Solid Edge part; units mm, degrees
sketch "Sketch1" plane through (0, 0, 0) normal (0, 0, 1) x (1, 0, 0)
  circle A0 centre (0, 0) radius 7.239
extrude "Protrusion1" add sketch "Sketch1" along normal blind 2.794
sketch "Sketch2" plane through (0, 0, 0) normal (0, 0, -1) x (1, 0, 0)
  line L0 (4.4626, 4.4626) -> (1.6334, 6.096)
  line L1 (1.6334, 6.096) -> (-1.6334, 6.096)
  line L2 (-1.6334, 6.096) -> (-4.4626, 4.4626)
  line L3 (-4.4626, 4.4626) -> (-6.096, 1.6334)
  line L4 (-6.096, 1.6334) -> (-6.096, -1.6334)
  line L5 (-6.096, -1.6334) -> (-4.4626, -4.4626)
  line L6 (-4.4626, -4.4626) -> (-1.6334, -6.096)
  line L7 (-1.6334, -6.096) -> (1.6334, -6.096)
  line L8 (1.6334, -6.096) -> (4.4626, -4.4626)
  line L9 (4.4626, -4.4626) -> (6.096, -1.6334)
  line L10 (6.096, -1.6334) -> (6.096, 1.6334)
  line L11 (6.096, 1.6334) -> (4.4626, 4.4626)
extrude "ExtrudedProtrusion_2" add sketch "Sketch2" along normal blind 10.922
sketch "Sketch3" plane through (0, 0, -10.922) normal (0, 0, -1) x (0.5, 0.866, 0)
  circle A0 centre (0, 0) radius 5.461
extrude "ExtrudedProtrusion_3" add sketch "Sketch3" along normal blind 10.16
sketch "Sketch4" plane through (0, 0, -21.082) normal (0, 0, -1) x (0, 1, 0)
  circle A0 centre (0, 0) radius 1.4
extrude "ExtrudedCutout_1" cut sketch "Sketch4" against normal blind 1.7575
Part model, mm, in its own coordinate system. A direction names the side the tool comes from. Coordinates: 2 decimals unless noted, no trailing zeros. Loops run counter-clockwise (first coordinate to the right, second up) from the corner with the lowest first, then second, coordinate; pieces in that order, holes last. Notation, with made-up numbers: (45, 87) -> (101, 87) arc R22 cw to (101, 110) -> close; hole circle Ø7 at (11.5, 57). An arc over 180 degrees is marked (long way). Use a Markdown table: item, result. Add a question column.
Item 1: Band-saw the part on C-C on z = 1. Write the cut outline in (x, y).
Item 2: Band-saw the part on D-D on y = -2.25. Write the cut outline in (x, z).
Item 3: Which spindle directions (+Z, -Z, +X, -X, +Y, -Y) get a long thin tool onto all of the face, cutting with end or side? Do faces 5 (the flat face through (-5.268, -3.068, -5.385)), 6 (the flat face through (-3.068, 5.268, -5.385)), 7 (the flat face through (0, 0, -19.324)). Say none if no direction does.
Item 4: Probe probe 1 along Z at (x, y) = (3.25, 4.75); probe 2 along Y at (x, z) = (1.5, -1.75). List the from-to ranges inside material, lowest first.
Item 5: Band-saw the part on A-A on x = 0. Write the cut outline in (y, z).
Item 6: Flat gauge pins, fed straight in: P1, Ø3.5, axis at x = -0.5, z = -7.5, coming from the +Y side; P2, Ø2.5, axis at y = -0.5, z = -5, coming from the -X side; P3, Ø3.5, axis at x = 0.5, z = -3, coming from the -Y side. Where does each tip first touch, or does it go through?
Item 7: Pull direction X, two halves, no side cores. Call faces 1 (the flat face through (-6.096, 0, -5)), 2 (the cylindrical face through (0.06, -1.4, -20.22)), 3 (the flat face through (3.03, 5.29, -5.38)), 4 (the flat face through (-1.1, -1.1, -21.082)): +X half, -X half, draft (parallel to the pull), parting line (faces both ways), or undercut.
Geometry says:
| question | item | result |
|---|---|---|
| 1 | outline | circle Ø14.48 at (0, 0) |
| 2 | outline | (-6.88, 0) -> (-5.74, 0) -> (-5.74, -10.92) -> (-4.98, -10.92) -> (-4.98, -21.08) -> (4.98, -21.08) -> (4.98, -10.92) -> (5.74, -10.92) -> (5.74, 0) -> (6.88, 0) -> (6.88, 2.79) -> (-6.88, 2.79) -> close |
| 3 | face 5 | -Z, -X, -Y |
| 3 | face 6 | -Z, -X, +Y |
| 3 | face 7 | -Z |
| 4 | probe 1 | -10.92 to 2.79 |
| 4 | probe 2 | -6.1 to 6.1 |
| 5 | outline | (-7.24, 0) -> (-6.1, 0) -> (-6.1, -10.92) -> (-5.46, -10.92) -> (-5.46, -21.08) -> (-1.4, -21.08) -> (-1.4, -19.32) -> (1.4, -19.32) -> (1.4, -21.08) -> (5.46, -21.08) -> (5.46, -10.92) -> (6.1, -10.92) -> (6.1, 0) -> (7.24, 0) -> (7.24, 2.79) -> (-7.24, 2.79) -> close |
| 6 | P1 | y = 6.1 |
| 6 | P2 | x = -6.1 |
| 6 | P3 | y = -6.1 |
| 7 | face 1 | -X half |
| 7 | face 2 | undercut |
| 7 | face 3 | +X half |
| 7 | face 4 | draft |
